Design review of the part built by this model. Coordinates are the model's own, in mm. A direction names the side the tool comes from. Round coordinates to 2 decimals unless told otherwise and drop trailing zeros. Loops run counter-clockwise (first coordinate to the right, second up) from the corner with the lowest first, then second, coordinate; pieces in that order, holes last. Notation, with made-up numbers: (61, 22.5) - (107, 22.5) arc R26 ccw to (107, 38.5) - close; hole circle Ø9 at (64.5, 1.25). An arc over 180 degrees is marked (long way). Use one line per item in the form item = value. Start each with the question number.
(1) Wall thickness on probe 1 along Z at (x, y) = (5, -6); probe 2 along Y at (x, z) = (10, 5.25) (3 decimals); probe 3 along X at (y, z) = (2, -6.25): over which ranges is each line inside the solid? List them lowest first. Write a range as [from, to].
(2) For pin 1 (4 mm diameter, centred on x = 22, z = 9.5, fed in from -Y) (3 decimals); pin 2 (1 mm diameter, centred on x = 15.5, y = 9.5, fed in from -Z); pin 3 (8 mm diameter, centred on x = -2, z = 10, fed in from +Y) (3 decimals), all flat-tipped, find the tip position at first contact; note any pin that passes through.
(3) We need section A-A, the plane y = 0. Write out the cut boundary in (x, z), then the cut area to 3 significant figures.
(4) We need section D-D, the plane x = -9. Write out the cut boundary in (y, z) (1 decimal).
(5) We need section B-B, the plane x = 16. Write out the cut boundary in (y, z) (1 decimal), then the cut area to 3 significant figures.
(6) The part is to be moulded in two halves that separate along Y. For faces 5 (the flat face through (-30.162, -6.5, -0.1)), 6 (the flat face through (-21, -9.525, -10)), 7 (the flat face through (22, 12.7, 4)), say which applies: released by +Y, released by -Y, zero draft, split by the parting line, or undercut.
(7) Machinability: for faces 1 (the flat face through (-21, 11.112, -3)), 2 (the cylindrical face through (-14.284, 0.14, 11.068)), 3 (the flat face through (30, -9.525, -7)), 4 (the cylindrical face through (27.45, -11.92, -1.03)), which of the approach directions +Z, -Z, +X, -X, +Y, -Y give a long, thin tool a straight path to every point of the face, cutting with its end or side? Answer none if there is none.
from build123d import *

# Parameters (mm, degrees)
F0_W      = 60.325
F0_H      = 15.875
F1_DEPTH  = 9.525
F3_DEPTH  = 3.175
F5_R      = 7.14375
F6_DEPTH  = 1.5875
F9_R      = 6.35
F10_DEPTH = 3.175
F11_R     = 2.54
F13_R     = 3.175
F14_DEPTH = 6.35


# Not quite as in the source:
# - a length typed as a fraction of an inch, garbled in the dataset ("3 / 203.2 mm" for 3/8 in), is restored
# - a feature names something its author has since deleted; it is built from what else it names
# - the program builds the solid bodies; features that only make, move or delete a surface that nothing else refers to are left out


with BuildPart() as f1:
    # F0 (on Front) → F1 (new body, symmetric)
    with BuildSketch(Plane.XZ):
        Rectangle(F0_W, F0_H)
    extrude(amount=F1_DEPTH, both=True)

    # F2 (on face) → F3 (join)
    with BuildSketch(Plane.XZ.offset(9.525)):
        with BuildLine():
            ThreePointArc((28.886391971, -7.9375), (29.8379434954, -5.6402514046), (30.1625, -3.175))
            ThreePointArc((30.1625, -3.175), (18.1722485954, 6.0254434954), (12.388608029, -7.9375))
            Line((12.388608029, -7.9375), (20.6375, -7.9375))
            Line((20.6375, -7.9375), (28.886391971, -7.9375))
        make_face()
        with BuildLine():
            Line((20.6375, -3.175), (20.6375, -7.9375))
            ThreePointArc((20.6375, -7.9375), (15.875, -3.175), (20.6375, 1.5875))
            Line((20.6375, 1.5875), (20.6375, -3.175))
        make_face(mode=Mode.SUBTRACT)
        with BuildLine():
            ThreePointArc((20.6375, 1.5875), (15.875, -3.175), (20.6375, -7.9375))
            Line((20.6375, -7.9375), (20.6375, -3.175))
            Line((20.6375, -3.175), (20.6375, 1.5875))
        make_face()
        with BuildLine():
            Line((20.6375, -7.9375), (12.388608029, -7.9375))
            ThreePointArc((12.388608029, -7.9375), (20.6375, -12.7), (28.886391971, -7.9375))
            Line((28.886391971, -7.9375), (20.6375, -7.9375))
        make_face()
    extrude(amount=F3_DEPTH)

    # F5 (on face) → F6 (cut)
    with BuildSketch(Plane.XZ.offset(12.7)):
        with Locations((20.6375, -3.175)):
            Circle(F5_R)
    extrude(amount=-F6_DEPTH, mode=Mode.SUBTRACT)


with BuildPart() as f7_1:
    # F7: instance of F1
    add(f1.part.mirror(Plane.YZ))


with BuildPart() as f8_1:
    # F8: instance of F1
    add(f1.part.mirror(Plane.XZ))


with BuildPart() as f8_2:
    # F8: instance of F7_1
    add(f7_1.part.mirror(Plane.XZ))


with BuildPart() as f1_1:
    add(f1.part)

    add(f7_1.part)  # F10 merges F7_1

    add(f8_1.part)  # F10 merges F8_1

    add(f8_2.part)  # F10 merges F8_2
    # F9 (on face) → F10 (join)
    with BuildSketch(Plane(origin=(-30.1625, 0, 0), x_dir=(0, -1, 0), z_dir=(-1, 0, 0))):
        Circle(F9_R)
    extrude(amount=F10_DEPTH)

    # F11
    f11_edges = [f1_1.edges().sort_by_distance(p)[0] for p in [
        (-33.3375, 6.35, 0),
    ]]
    fillet(f11_edges, radius=F11_R)


with BuildPart() as f12_1:
    # F12: instance of F1
    add(f1_1.part.mirror(Plane.YZ))


with BuildPart() as f1_2:
    add(f1_1.part)

    add(f12_1.part)  # F14 merges F12_1
    # F13 (on face) → F14 (join)
    with BuildSketch(Plane.XY.offset(7.9375)):
        with Locations((-11.1125, 0)):
            Circle(F13_R)
        with Locations((11.1125, 0)):
            Circle(F13_R)
    extrude(amount=F14_DEPTH)


solid = f1_2.part
Data:
q1.probe_1 = [-7.94, 7.94]
q1.probe_2 = [-9.525, 9.525]
q1.probe_3 = [-30.16, 30.16]
q2.pin_1 = -9.525
q2.pin_2 = -11.49
q2.pin_3 = 9.525
q3.outline = (-33.34, -3.81) arc R2.54 ccw to (-30.8, -6.35) - (-30.16, -6.35) - (-30.16, -7.94) - (30.16, -7.94) - (30.16, -6.35) - (30.8, -6.35) arc R2.54 ccw to (33.34, -3.81) - (33.34, 3.81) arc R2.54 ccw to (30.8, 6.35) - (30.16, 6.35) - (30.16, 7.94) - (14.29, 7.94) - (14.29, 14.29) - (7.94, 14.29) - (7.94, 7.94) - (-7.94, 7.94) - (-7.94, 14.29) - (-14.29, 14.29) - (-14.29, 7.94) - (-30.16, 7.94) - (-30.16, 6.35) - (-30.8, 6.35) arc R2.54 ccw to (-33.34, 3.81) - close
q3.area = 1,110 mm^2
q4.outline = (-9.5, -7.9) - (9.5, -7.9) - (9.5, 7.9) - (2.4, 7.9) - (2.4, 14.3) - (-2.4, 14.3) - (-2.4, 7.9) - (-9.5, 7.9) - close
q5.outline = (-12.7, -11.5) - (-9.5, -11.5) - (-9.5, -7.9) - (9.5, -7.9) - (9.5, -11.5) - (12.7, -11.5) - (12.7, -8.6) - (11.1, -8.6) - (11.1, 2.3) - (12.7, 2.3) - (12.7, 5.1) - (9.5, 5.1) - (9.5, 7.9) - (-9.5, 7.9) - (-9.5, 5.1) - (-12.7, 5.1) - (-12.7, 2.3) - (-11.1, 2.3) - (-11.1, -8.6) - (-12.7, -8.6) - close
q5.area = 374 mm^2
q6.face_5 = zero draft
q6.face_6 = undercut
q6.face_7 = released by +Y
q7.face_1 = +Y
q7.face_2 = +Z
q7.face_3 = -Z, +X, -Y
q7.face_4 = -Y
